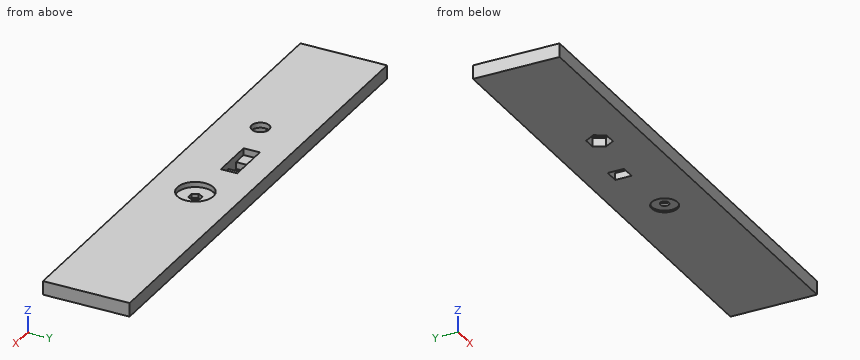
from build123d import *

# Parameters (mm, degrees)
SKETCH1_W                  = 571.5
SKETCH1_H                  = 100.8
BOSS_EXTRUDE1_DEPTH        = 8
SKETCH4_R                  = 7.5
CUT_EXTRUDE3_DEPTH         = 2
SKETCH5_R                  = 5
CUT_EXTRUDE4_DEPTH         = 581.490215249
CUT_EXTRUDE5_DEPTH         = 11
SKETCH9_R                  = 10.2
POWER_AND_USB_CABLES_DEPTH = 581.541893406
SKETCH10_R                 = 21
CUT_EXTRUDE6_DEPTH         = 6
CUT_EXTRUDE8_DEPTH         = 10
CUT_EXTRUDE9_DEPTH         = 581.541893406
CUT_EXTRUDE9_DEPTH_BACK    = 581.541893406
SKETCH13_W                 = 16.7
SKETCH13_H                 = 19
SKETCH14_W                 = 50.4
SKETCH14_H                 = 19
CUT_EXTRUDE10_DEPTH        = 8
SKETCH15_R                 = 15
CUT_EXTRUDE11_DEPTH        = 2


with BuildPart() as part:
    # Sketch1 → Boss-Extrude1 (new, symmetric)
    with BuildSketch(Plane.XY):
        with Locations((285.75, 50.4)):
            Rectangle(SKETCH1_W, SKETCH1_H)
    extrude(amount=BOSS_EXTRUDE1_DEPTH, both=True)

    # Sketch4 → Cut-Extrude3 (cut)
    with BuildSketch(Plane(origin=(0, 0, -8), x_dir=(-1, 0, 0), z_dir=(0, 0, -1))):
        with Locations((-330.123617772, 50.8)):
            Circle(SKETCH4_R)
    extrude(amount=-CUT_EXTRUDE3_DEPTH, mode=Mode.SUBTRACT)

    # Sketch5 → Cut-Extrude4 (cut, through all)
    with BuildSketch(Plane(origin=(0, 0, -6), x_dir=(-1, 0, 0), z_dir=(0, 0, -1))):
        with Locations((-330.123617772, 50.8)):
            Circle(SKETCH5_R)
    extrude(amount=-CUT_EXTRUDE4_DEPTH, mode=Mode.SUBTRACT)

    # Sketch6 → Cut-Extrude5 (cut)
    with BuildSketch(Plane.XY.offset(8)):
        Polygon((337.467513196, 50.8), (333.795565484, 57.16), (326.45167006, 57.16), (322.779722348, 50.8), (326.45167006, 44.44), (333.795565484, 44.44), align=None)
    extrude(amount=-CUT_EXTRUDE5_DEPTH, mode=Mode.SUBTRACT)

    # Sketch9 → power and usb cables (cut, through all)
    with BuildSketch(Plane.XY.offset(8)):
        with Locations((177.536724471, 46.600039321)):
            Circle(SKETCH9_R)
    extrude(amount=-POWER_AND_USB_CABLES_DEPTH, mode=Mode.SUBTRACT)

    # Sketch10 → Cut-Extrude6 (cut)
    with BuildSketch(Plane.XY.offset(8)):
        with Locations((330.16394587, 50.821844921)):
            Circle(SKETCH10_R)
    extrude(amount=-CUT_EXTRUDE6_DEPTH, mode=Mode.SUBTRACT)

    # Sketch12 → Cut-Extrude8 (cut)
    with BuildSketch(Plane(origin=(0, 0, -8), x_dir=(-1, 0, 0), z_dir=(0, 0, -1))):
        Polygon((-163.68031801, 46.600039321), (-170.608521241, 58.600039321), (-184.464927701, 58.600039321), (-191.393130932, 46.600039321), (-184.464927701, 34.600039321), (-170.608521241, 34.600039321), align=None)
    extrude(amount=-CUT_EXTRUDE8_DEPTH, mode=Mode.SUBTRACT)

    # Sketch13 → Cut-Extrude9 (cut, two sides: drawn at the far end of the back side and taken through both)
    with BuildSketch(Plane(origin=(0, 0, -8), x_dir=(-1, 0, 0), z_dir=(0, 0, -1)).offset(-CUT_EXTRUDE9_DEPTH_BACK)):
        with Locations((-250.2, 61.3)):
            Rectangle(SKETCH13_W, SKETCH13_H)
    extrude(amount=CUT_EXTRUDE9_DEPTH + CUT_EXTRUDE9_DEPTH_BACK, mode=Mode.SUBTRACT)

    # Sketch14 → Cut-Extrude10 (cut)
    with BuildSketch(Plane.XY.offset(8)):
        with Locations((250.2, 61.3)):
            Rectangle(SKETCH14_W, SKETCH14_H)
    extrude(amount=-CUT_EXTRUDE10_DEPTH, mode=Mode.SUBTRACT)

    # Sketch15 → Cut-Extrude11 (cut)
    with BuildSketch(Plane(origin=(0, 0, -8), x_dir=(-1, 0, 0), z_dir=(0, 0, -1))):
        with Locations((-330.16394587, 50.821844921)):
            Circle(SKETCH15_R)
    extrude(amount=-CUT_EXTRUDE11_DEPTH, mode=Mode.SUBTRACT)


solid = part.part
Model file for the job. Use its own axes, mm. Round coordinates to 2 decimals unless told otherwise and drop trailing zeros. Loops run counter-clockwise (first coordinate to the right, second up) from the corner with the lowest first, then second, coordinate; pieces in that order, holes last. Notation, with made-up numbers: M 36,37.5 L 81,37.5 A20 ccw 81,55.5 Z; hole C 71.5,56 d7. An arc over 180 degrees is marked long. One line per question, with ' | ' between items.
1) Drill centre lines: line 1 along X through (y, z) = (58.5, 0.25); line 2 along X through (y, z) = (54.5, 3); line 3 along X through (y, z) = (61, 7.5). Where is each one in solid material? Low to high.
Solved:
line 1: x = 0 to 170.55, 184.52 to 225, 275.4 to 571.5 | line 2: x = 0 to 171.08, 183.99 to 225, 275.4 to 309.49, 350.84 to 571.5 | line 3: x = 0 to 225, 275.4 to 311.8, 348.53 to 571.5
2) Flat gauge pins, fed straight in: pin 1 (4 mm diameter, centred on x = 331.5, y = 51.5, fed in from +Z); pin 2 (21 mm diameter, centred on x = 337.5, y = 50, fed in from +Z). Where does each tip first touch, or does it go through?
Solved:
pin 1: passes through | pin 2: stops at z = 2
3) Band-saw the part on A-A (x = 235.5). Give the cut face in (y, z), then the cut area to 3 significant figures.
Solved:
outline: M 0,-8 L 100.8,-8 L 100.8,8 L 70.8,8 L 70.8,0 L 51.8,0 L 51.8,8 L 0,8 Z | area: 1,460 mm²
